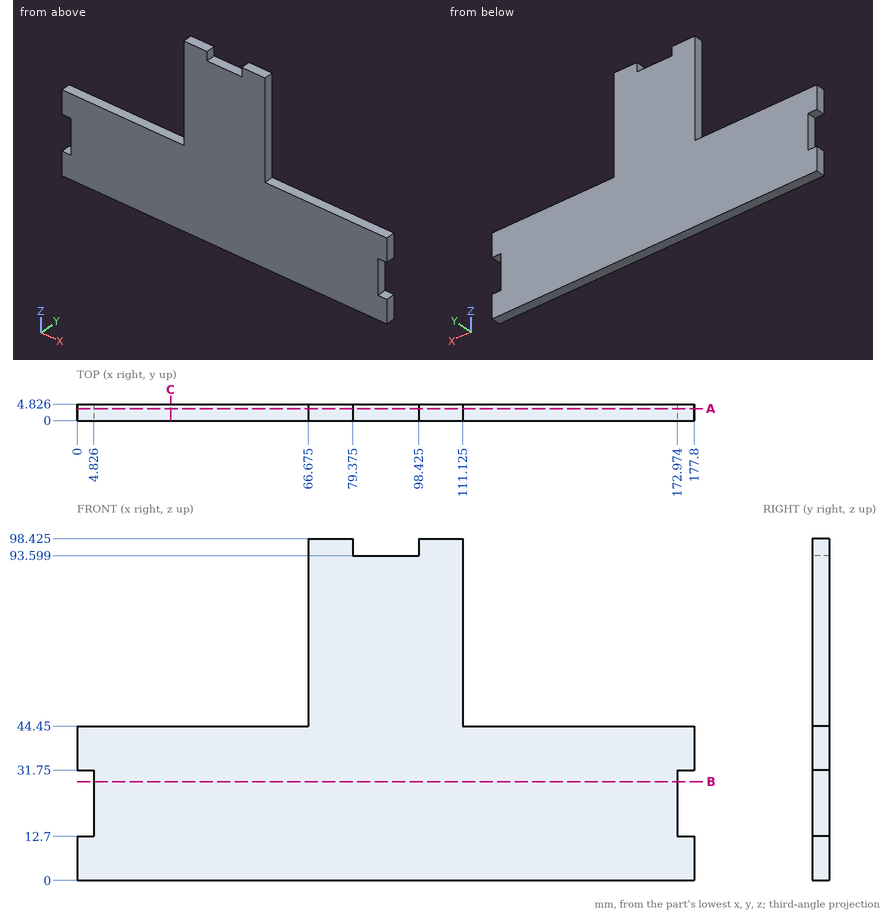
Job drawing, mm, ordinate dimensions from the low corner. One solid piece. Give positions to 0.01 mm unless a question says otherwise; leave off trailing zeros. Loops run counter-clockwise (first coordinate to the right, second up) from the corner with the lowest first, then second, coordinate; pieces in that order, holes last. Notation, with made-up numbers: (42.25, 77) -> (101.25, 77) arc R33 ccw to (101.25, 105) -> close; hole circle Ø3 at (82.25, 73). An arc over 180 degrees is marked (long way). Use a Markdown table: item, result. Add a question column.
(1) Drop flat-ended pins along their axis: pin 1 Ø2.5 at (y, z) = (3.5, 96.5) entering from -X (3 decimals); pin 2 Ø1.5 at (y, z) = (3, 40.5) entering from -X; pin 3 Ø2.5 at (x, y) = (144, 3.5) entering from +Z; pin 4 Ø2.5 at (y, z) = (1.5, 79) entering from +X (3 decimals). Give the stop position or say it passes through.
(2) Slice it at B-B on z = 28.5. List the corners of the cut face in (x, y).
(3) Slice it at C-C on x = 27. List the corners of the cut face in (y, z), and give its area (3 significant figures).
(4) Wall check: line 1 along X through (y, z) = (4.4, 14); line 2 along Z through (x, y) = (89.5, 0.95); line 3 along Z through (x, y) = (132.5, 0.5). Give the ranges that are in metal, low to high.
(5) Slice it at A-A on y = 3.5. List the corners of the cut face in (x, z) (3 decimals).
Filled sheet:
| question | item | result |
|---|---|---|
| 1 | pin 1 | x = 66.675 |
| 1 | pin 2 | x = 0 |
| 1 | pin 3 | z = 44.45 |
| 1 | pin 4 | x = 111.125 |
| 2 | outline | (4.83, 0) -> (172.97, 0) -> (172.97, 4.83) -> (4.83, 4.83) -> close |
| 3 | outline | (0, 0) -> (4.83, 0) -> (4.83, 44.45) -> (0, 44.45) -> close |
| 3 | area | 215 mm2 |
| 4 | line 1 | 4.83 to 172.97 |
| 4 | line 2 | 0 to 93.6 |
| 4 | line 3 | 0 to 44.45 |
| 5 | outline | (0, 0) -> (177.8, 0) -> (177.8, 12.7) -> (172.974, 12.7) -> (172.974, 31.75) -> (177.8, 31.75) -> (177.8, 44.45) -> (111.125, 44.45) -> (111.125, 98.425) -> (98.425, 98.425) -> (98.425, 93.599) -> (79.375, 93.599) -> (79.375, 98.425) -> (66.675, 98.425) -> (66.675, 44.45) -> (0, 44.45) -> (0, 31.75) -> (4.826, 31.75) -> (4.826, 12.7) -> (0, 12.7) -> close |
